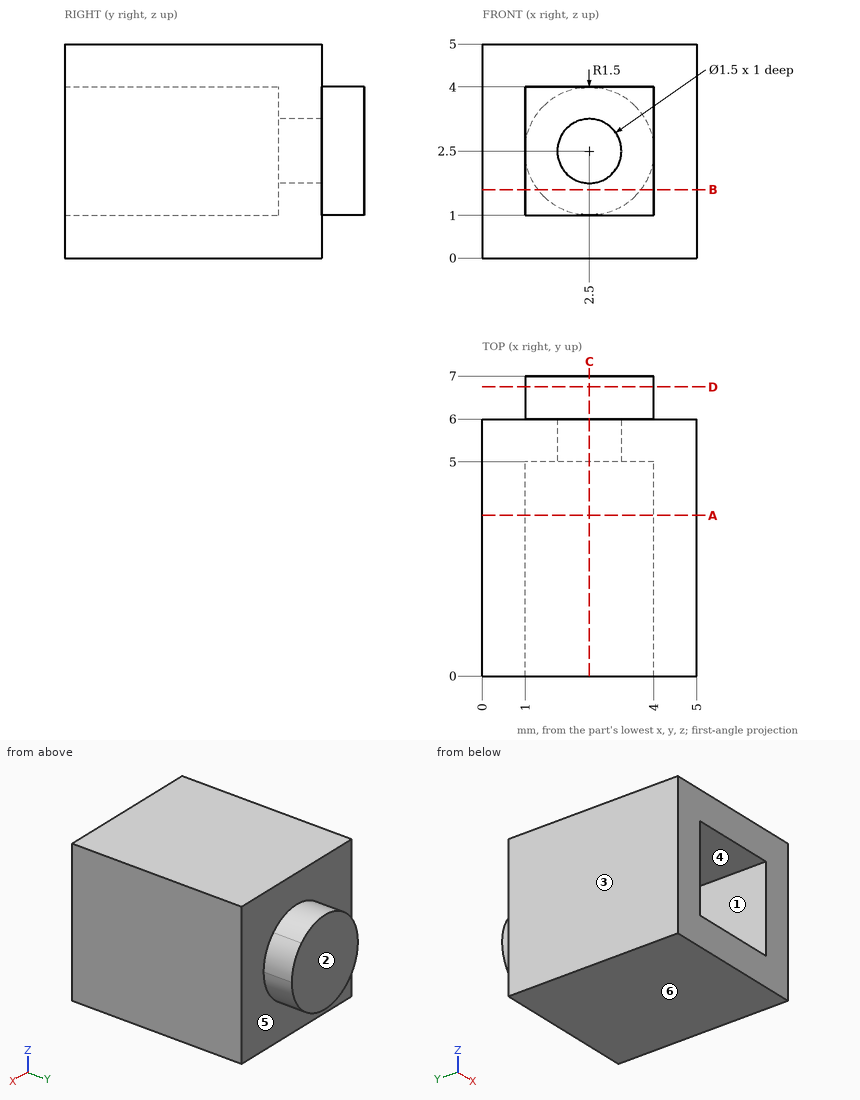
Here's the drawing with two shaded views (mm, measured from the low corner). I have some questions. A direction names the side the tool comes from. Give positions to 0.01 mm unless a question says otherwise; leave off trailing zeros. Write each loop counter-clockwise with the first axis right and the second up, starting at its lowest first coordinate (ties: lowest second). Pieces come first, ordered by that corner, then holes. Notation, with made-up numbers: (71.5, 69.25) - (106.5, 69.25) arc R4 ccw to (106.5, 74.25) - close; hole circle Ø1 at (13, 19). An arc over 180 degrees is marked (long way). One line per item, written item: value. Start each with the question number.
Item 1: Imagine slicing it at A-A, the plane y = 3.75. List the corners of the cut face in (x, z) for me, and give its area (3 significant figures).
Item 2: If we mould it in two halves opening along X, with no side actions, what happens to the marked faces 1, 2 and 3? For each: +X half, -X half, draft (parallel to the pull), parting line (faces both ways), or undercut.
Item 3: Please list where these lines run through material, in increasing order: line 1 (X direction, y = 2.75, z = 2.75); line 2 (Z direction, x = 2.5, y = 5.75). Write a range as from..to.
Item 4: Which directions (+Z, -Z, +X, -X, +Y, -Y) give clear straight access to the entire face, cutting with the end or side of a thin tool? Please do the marked faces 4, 5 and 6.
Item 5: I'm going to push a flat-ended pin straight in: pin 1 (1.5 mm diameter, centred on x = 2, z = 3, fed in from -Y). Where does the tip first touch, or does it pass through?
Item 6: Imagine slicing it at D-D, the plane y = 6.75. List the corners of the cut face in (x, z) for me, and give its area (3 significant figures).
Item 7: Imagine slicing it at C-C, the plane x = 2.5. List the corners of the cut face in (y, z) for me, and give its area (3 significant figures).
Item 8: Imagine slicing it at B-B, the plane z = 1.6. List the corners of the cut face in (x, y) for me.
Geometry says:
1. outline: (0, 0) - (5, 0) - (5, 5) - (0, 5) - close; hole (1, 1) - (4, 1) - (4, 4) - (1, 4) - close
1. area: 16.0 mm^2
2. face 1: undercut
2. face 2: draft
2. face 3: -X half
3. line 1: 0..1, 4..5
3. line 2: 0..1.75, 3.25..5
4. face 4: -Y
4. face 5: +Y
4. face 6: -Z, +X, -X, +Y, -Y
5. pin 1: y = 5
6. outline: circle Ø3 at (2.5, 2.5)
6. area: 7.07 mm^2
7. outline: (0, 0) - (6, 0) - (6, 1) - (7, 1) - (7, 4) - (6, 4) - (6, 5) - (0, 5) - (0, 4) - (5, 4) - (5, 3.25) - (6, 3.25) - (6, 1.75) - (5, 1.75) - (5, 1) - (0, 1) - close
7. area: 16.5 mm^2
8. outline: (0, 0) - (1, 0) - (1, 5) - (4, 5) - (4, 0) - (5, 0) - (5, 6) - (3.7, 6) - (3.7, 7) - (1.3, 7) - (1.3, 6) - (0, 6) - close
